Read the model definition and answer for the solid it produces. Units are mm, in the model's axes. A direction names the side the tool comes from. Coordinates: 2 decimals unless noted, no trailing zeros. Order: outer loops, then holes, each group sorted by start corner. A loop starts at its lowest first (then second) coordinate and runs counter-clockwise, first axis right, second up.
```python
from build123d import *

# Parameters (mm, degrees)
CROQUIS3_R              = 31.75
SALIENTE_EXTRUIR3_DEPTH = 97
CROQUIS4_R              = 7
CORTAR_EXTRUIR1_DEPTH   = 107.888376356
CROQUIS8_R              = 2.5
CORTAR_EXTRUIR6_DEPTH   = 107.888376356
MATRIZC1_COUNT          = 6
CUT_EXTRUDE1_START      = -4
SKETCH1_R               = 31.75
SKETCH1_R_2             = 14.25
CUT_EXTRUDE1_DEPTH      = 4


with BuildPart() as part:
    # Croquis3 → Saliente-Extruir3 (new body)
    with BuildSketch(Plane.XY):
        with Locations(Location((0, 0, 0), (0, 0, 180))):
            Circle(CROQUIS3_R)
    extrude(amount=SALIENTE_EXTRUIR3_DEPTH)

    # Croquis4 → Cortar-Extruir1 (cut, through all)
    with BuildSketch(Plane.XY.offset(97)):
        Circle(CROQUIS4_R)
    extrude(amount=-CORTAR_EXTRUIR1_DEPTH, mode=Mode.SUBTRACT)

    # Croquis8 → Cortar-Extruir6 (cut, through all)
    with BuildSketch(Plane.XY.offset(97)):
        with Locations((0, 23.8)):
            Circle(CROQUIS8_R)
    cortar_extruir6 = extrude(amount=-CORTAR_EXTRUIR6_DEPTH, mode=Mode.SUBTRACT)

    # MatrizC1: Cortar-Extruir6 ×6 about axis
    matrizc1_axis = Axis((0, 0, 0), (0, 0, 1))
    for i in range(1, MATRIZC1_COUNT):
        add(cortar_extruir6.rotate(matrizc1_axis, i * 360 / MATRIZC1_COUNT), mode=Mode.SUBTRACT)

    # Sketch1 → Cut-Extrude1 (cut)
    with BuildSketch(Plane.XY.offset(97).offset(CUT_EXTRUDE1_START)):
        with Locations(Location((0, 0, 0), (0, 0, 180))):
            Circle(SKETCH1_R)
        Circle(SKETCH1_R_2, mode=Mode.SUBTRACT)
    cut_extrude1 = extrude(amount=CUT_EXTRUDE1_DEPTH, mode=Mode.SUBTRACT)

    # Mirror1: Cut-Extrude1 across plane
    add(cut_extrude1.mirror(Plane.XY.offset(48.5)), mode=Mode.SUBTRACT)


solid = part.part
```
1) Flat-ended cylindrical pins translate along their axes: pin 1 Ø10 at (x, z) = (14.5, 42) entering from -Y; pin 2 Ø6 at (x, y) = (23, 1.5) entering from -Z; pin 3 Ø6 at (x, z) = (-0.5, 83.5) entering from +Y. Find the tip coordinate at first contact, or state that the pin passes through.
A:
pin 1: stops at y = -30.3
pin 2: stops at z = 4
pin 3: stops at y = 31.75
2) Which of the six approach directions +Z, -Z, +X, -X, +Y, -Y give full straight-line access (tool end or side, diameter ignored) to faces 1 (the cylindrical face through (-18.627, 13.421, 49.123)), 2 (the cylindrical face through (13.163, -5.458, 94.972))?
A:
face 1: +Z, -Z
face 2: +Z
3) A cutting plane is placed at D-D, the plane y = 11.9. Determine the outline of the cut face in (x, z).
A:
outline: (-29.44, 4) - (-23.11, 4) - (-23.11, 93) - (-29.44, 93) - close; (-18.11, 4) - (-7.84, 4) - (-7.84, 0) - (7.84, 0) - (7.84, 4) - (18.11, 4) - (18.11, 93) - (7.84, 93) - (7.84, 97) - (-7.84, 97) - (-7.84, 93) - (-18.11, 93) - close; (23.11, 4) - (29.44, 4) - (29.44, 93) - (23.11, 93) - close
4) A cutting plane is placed at C-C, the plane z = 17.5. Determine the outline of the cut face in (x, y).
A:
outline: circle Ø63.5 at (0, 0); hole circle Ø5 at (-20.61, -11.9); hole circle Ø5 at (-20.61, 11.9); hole circle Ø14 at (0, 0); hole circle Ø5 at (0, -23.8); hole circle Ø5 at (0, 23.8); hole circle Ø5 at (20.61, -11.9); hole circle Ø5 at (20.61, 11.9)
5) Determine the mould class of faces 3 (the cylindrical face through (-19.27, -9.79, 49.12)), 4 (the cylindrical face through (13.163, -5.458, 2.028)), 5 (the flat face through (-14, 7, 4)) for opening direction Y: pulls with the +Y half, pulls with the -Y half, needs draft (parallel to the pull), parting line crosses it, or undercut.
A:
face 3: undercut
face 4: parting line crosses it
face 5: needs draft
6) Straight lines are drawn through the part: line 1 (Y direction, x = 0, z = 37); line 2 (X direction, y = 11, z = 23); line 3 (X direction, y = 13, z = 47.5). For each, find the intervals that lie inside material, in ascending order.
A:
line 1: y = -31.75 to -26.3, -21.3 to -7, 7 to 21.3, 26.3 to 31.75
line 2: x = -29.78 to -22.94, -18.28 to 18.28, 22.94 to 29.78
line 3: x = -28.97 to -22.86, -18.37 to 18.37, 22.86 to 28.97
7) A cutting plane is placed at A-A, the plane x = 0. Determine the outline of the cut face in (y, z).
A:
outline: (-31.75, 4) - (-26.3, 4) - (-26.3, 93) - (-31.75, 93) - close; (-21.3, 4) - (-14.25, 4) - (-14.25, 0) - (-7, 0) - (-7, 97) - (-14.25, 97) - (-14.25, 93) - (-21.3, 93) - close; (7, 0) - (14.25, 0) - (14.25, 4) - (21.3, 4) - (21.3, 93) - (14.25, 93) - (14.25, 97) - (7, 97) - close; (26.3, 4) - (31.75, 4) - (31.75, 93) - (26.3, 93) - close
8) A cutting plane is placed at B-B, the plane y = -23.8. Determine the outline of the cut face in (x, z), and give its area (3 significant figures).
A:
outline: (-21.01, 4) - (-2.5, 4) - (-2.5, 93) - (-21.01, 93) - close; (2.5, 4) - (21.01, 4) - (21.01, 93) - (2.5, 93) - close
area: 3,300 mm2
